Input: part model. Units: mm. Frame: model coordinates. Give positions to 0.01 mm unless a question says otherwise; leave off trailing zeros. Loops run counter-clockwise (first coordinate to the right, second up) from the corner with the lowest first, then second, coordinate; pieces in that order, holes last. Notation, with made-up numbers: M -36.75,43.25 L 19.25,43.25 A27 ccw 19.25,80.25 Z; hole C 31.25,78 d7. An arc over 180 degrees is marked long. Use CSV: the item, a comma, the result in double quotes. Start each with the question number.
Q1. Pin query (flat end, axial travel): pin 1 (3 mm diameter, centred on y = -8, z = -12.5, fed in from -X). Return the tip coordinate at first contact, or that it passes through.
Q2. Section C-C, the plane y = -5.5. Output: boundary loops of the cut face in (x, z), plus the area to 3 significant figures.
Q3. Material intervals for line 1 along X through (y, z) = (-0.25, 46); line 2 along X through (y, z) = (-0.75, 37); line 3 along Y through (x, z) = (-123.5, 33.5), sorted ascending.
from build123d import *

# Parameters (mm, degrees)
F0_W     = 115
F0_H     = 121.7650999273
F1_DEPTH = 10
F2_SIZE2 = 8.888878
F2_SIZE  = 9.99999
F3_SIZE2 = 9.99999
F3_SIZE  = 8.888878


# Not quite as in the source:
# - a fillet or chamfer is up to 0.001 mm smaller than in the source, because OpenCascade refuses the exact size


with BuildPart() as f1:
    # F0 (on Front) → F1 (new body)
    with BuildSketch(Plane.XZ):
        with Locations((-35.6102311611, 0.0679380756)):
            Rectangle(F0_W, F0_H)
        Polygon((-93.1102311611, -60.814611888), (-93.1102311611, 60.9504880392), (-134.7733613184, 60.9504880392), align=None)
        Polygon((63.5528989962, 60.9504880392), (21.8897688389, 60.9504880392), (21.8897688389, -60.814611888), align=None)
    extrude(amount=F1_DEPTH)

    # F2 (size 10 and 8.888888 in the source; OpenCascade refuses exactly that, so slightly less here)
    f2_edges = [f1.edges().sort_by_distance(p)[0] for p in [
        (-113.941796, 0, 0.067938),
    ]]
    f2_side = f1.faces().sort_by_distance((-113.941796, -5, 0.067938))[0]
    chamfer(f2_edges, length=F2_SIZE, length2=F2_SIZE2, reference=f2_side)

    # F3 (size 8.888888 and 10 in the source; OpenCascade refuses exactly that, so slightly less here)
    f3_edges = [f1.edges().sort_by_distance(p)[0] for p in [
        (42.721334, 0, 0.067938),
    ]]
    f3_side = f1.faces().sort_by_distance((-30.912828, 0, 5.809289))[0]
    chamfer(f3_edges, length=F3_SIZE, length2=F3_SIZE2, reference=f3_side)


solid = f1.part
A:
1,pin 1,"x = -109.26"
2,outline,"M -130.55,60.95 L -88.88,-60.81 L 17.66,-60.81 L 59.33,60.95 Z"
2,area,"18,000 mm^2"
3,line 1,"-120.5 to 49.28"
3,line 2,"-117.89 to 46.67"
3,line 3,"-10 to -8"
